```python
from build123d import *

# Parameters (mm, degrees)
CUT_EXTRUDE1_DEPTH = 7.62
CIRPATTERN1_COUNT  = 3


with BuildPart() as part:
    # Sketch1 → Revolve1 (revolve)
    with BuildSketch(Plane.XY, mode=Mode.PRIVATE) as revolve1_sk:
        Polygon((15.248535153, 18.161), (2.548535153, 18.161), (2.548535153, 16.891), (193.048535153, 16.891), (193.048535153, 19.431), (15.248535153, 19.431), align=None)
    revolve(revolve1_sk.sketch.rotate(Axis((0, 0, 0), (1, 0, 0)), 90), axis=Axis((0, 0, 0), (1, 0, 0)))

    # Sketch2 → Cut-Extrude1 (cut)
    with BuildSketch(Plane(origin=(0, 19.431, 0), x_dir=(1, 0, 0), z_dir=(0, 1, 0))):
        with BuildLine():
            Line((26.9875, 2.54), (26.9875, -2.54))
            ThreePointArc((26.9875, -2.54), (25.4, -4.1275), (23.8125, -2.54))
            Line((23.8125, -2.54), (23.8125, 2.54))
            ThreePointArc((23.8125, 2.54), (25.4, 4.1275), (26.9875, 2.54))
        make_face()
    cut_extrude1 = extrude(amount=-CUT_EXTRUDE1_DEPTH, mode=Mode.SUBTRACT)

    # CirPattern1: Cut-Extrude1 ×3 about axis
    cirpattern1_axis = Axis((0, 0, 0), (-1, 0, 0))
    for i in range(1, CIRPATTERN1_COUNT):
        add(cut_extrude1.rotate(cirpattern1_axis, i * 360 / CIRPATTERN1_COUNT), mode=Mode.SUBTRACT)


solid = part.part
```
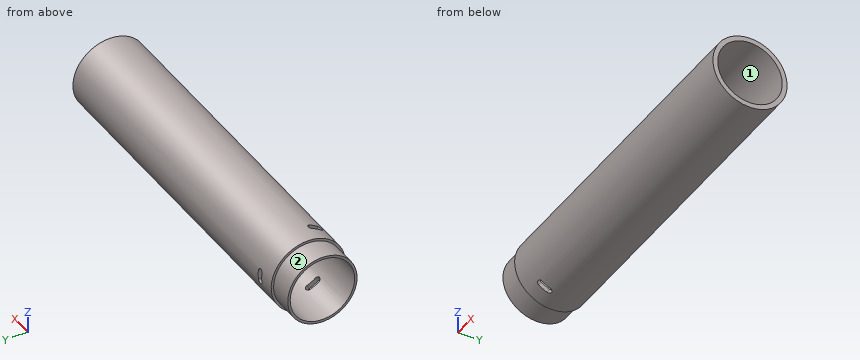
Part model, mm, in its own coordinate system. Face numbers are marked on the shaded views. Round coordinates to 2 decimals unless told otherwise and drop trailing zeros. Write each loop counter-clockwise with the first axis right and the second up, starting at its lowest first coordinate (ties: lowest second). Pieces come first, ordered by that corner, then holes. Notation, with made-up numbers: M -10.5,32 L 48.5,32 A21 ccw 48.5,60 Z; hole C 4.25,31.5 d5. An arc over 180 degrees is marked long. One line per question, with ' | ' between items.
(1) Saw through at D-D on x = 92. Write the cut outline in (y, z), then the cut area to 3 significant figures.
Answer key:
outline: C 0,0 d38.86; hole C 0,0 d33.78 | area: 290 mm^2
(2) Saw through at C-C on x = 25.4. Write the cut outline in (y, z), then the cut area to 3 significant figures.
Answer key:
outline: M -13.07,-14.38 L -11.76,-12.12 A16.89 cw -11.76,12.12 L -13.07,14.38 A19.43 ccw Z; M -5.92,-18.51 A19.43 ccw 18.99,-4.13 L 16.38,-4.13 A16.89 cw -4.61,-16.25 Z; M -5.92,18.51 L -4.61,16.25 A16.89 cw 16.38,4.13 L 18.99,4.13 A19.43 ccw Z | area: 226 mm^2
(3) Probe line 1 along Y through (x, z) = (44.5, 0); line 2 along X through (y, z) = (18, -2); line 3 along Z through (x, y) = (178, 14.5). List the from-to ranges inside material, lowest first.
Answer key:
line 1: y = -19.43 to -16.89, 16.89 to 19.43 | line 2: x = 2.55 to 23.81, 26.99 to 193.05 | line 3: z = -12.93 to -8.66, 8.66 to 12.93
(4) Saw through at B-B on z = -9. Write the cut outline in (x, y), then the cut area to 3 significant figures.
Answer key:
outline: M 2.55,-15.77 L 15.25,-15.77 L 15.25,-17.22 L 193.05,-17.22 L 193.05,-14.29 L 2.55,-14.29 Z; M 2.55,14.29 L 193.05,14.29 L 193.05,17.22 L 15.25,17.22 L 15.25,15.77 L 2.55,15.77 Z | area: 1,080 mm^2
(5) Pin check, flat tips, straight feed: pin 1 (5 mm diameter, centred on x = 101.5, y = 10.5, fed in from -Z); pin 2 (1 mm diameter, centred on x = 40.5, y = -10.5, fed in from +Z); pin 3 (4 mm diameter, centred on x = 153, z = -6.5, fed in from -Y); pin 4 (8 mm diameter, centred on y = 8.5, z = 5.5, fed in from +X). Stop position of each tip, or through.
Answer key:
pin 1: stops at z = -17.71 | pin 2: stops at z = 16.66 | pin 3: stops at y = -18.9 | pin 4: passes through
(6) Saw through at A-A on y = 4.5. Write the cut outline in (x, z), then the cut area to 3 significant figures.
Answer key:
outline: M 2.55,-17.59 L 15.25,-17.59 L 15.25,-18.9 L 193.05,-18.9 L 193.05,-16.28 L 2.55,-16.28 Z; M 2.55,16.28 L 193.05,16.28 L 193.05,18.9 L 15.25,18.9 L 15.25,17.59 L 2.55,17.59 Z | area: 966 mm^2
(7) Two-plate mould, pull along Y, no slides. Class the marked faces 1 and 2: released by +Y, released by -Y, zero draft, split by the parting line, or undercut.
Answer key:
face 1: undercut | face 2: split by the parting line
